The drawing under review shows one solid part. Ordinate dimensions are in mm from its lowest x, y, z. Coordinates: 2 decimals unless noted, no trailing zeros. Write each loop counter-clockwise with the first axis right and the second up, starting at its lowest first coordinate (ties: lowest second). Pieces come first, ordered by that corner, then holes.
Q1. Clearance check with flat-ended pins moving along their axes: pin 1 Ø5 at (y, z) = (41.5, 1.5) entering from +X; pin 2 Ø3 at (x, y) = (7, 49) entering from -Z; pin 3 Ø1.5 at (x, y) = (9.5, 47.5) entering from -Z. State where each tip first meets the part, or that it passes through.
Q2. Add section A-A, the plane z = 6.4. Give the boundary of the cut face in (x, y), plus the area to 3 significant figures.
Q3. The part is to be moulded in two halves that separate along Z. For the marked faces 1 and 2, say which applies: +Z half, -Z half, draft (parallel to the pull), parting line (faces both ways), or undercut.
Q4. To check wall thickness, follow probe 1 along X at (y, z) = (54, 6.5); probe 2 along Y at (x, z) = (1.5, 8). State the ranges of each line that lie inside material, in increasing order.
Q5. Add section B-B, the plane y = 60. Give the boundary of the cut face in (x, z).
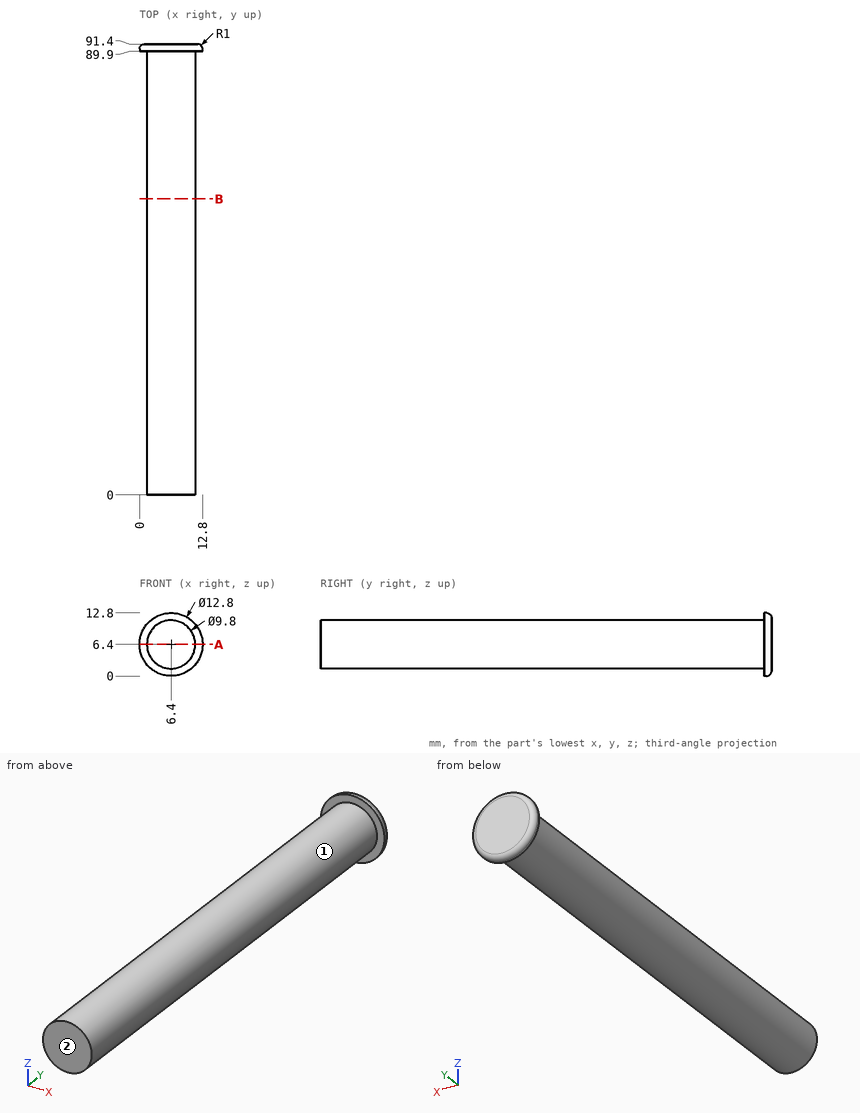
Here are the results:
1. pin 1: stops at x = 10.67
1. pin 2: stops at z = 1.5
1. pin 3: stops at z = 2.1
2. outline: (0, 89.9) - (1.5, 89.9) - (1.5, 0) - (11.3, 0) - (11.3, 89.9) - (12.8, 89.9) - (12.8, 90.4) arc R1 ccw to (11.8, 91.4) - (1, 91.4) arc R1 ccw to (0, 90.4) - close
2. area: 900 mm2
3. face 1: parting line
3. face 2: draft
4. probe 1: x = 1.5 to 11.3
4. probe 2: y = 89.9 to 91.4
5. outline: circle Ø9.8 at (6.4, 6.4)
